Verification items for the finished model (mm, model axes). A direction names the side the tool comes from. Coordinates: 2 decimals unless noted, no trailing zeros. Order: outer loops, then holes, each group sorted by start corner. A loop starts at its lowest first (then second) coordinate and runs counter-clockwise, first axis right, second up. Notation, with made-up numbers: (4, 65) -> (50, 65) arc R35 ccw to (50, 102) -> close; hole circle Ø9 at (-26.75, 35). An arc over 180 degrees is marked (long way). Use CSV: the item, a comma, the result in double quotes. Start each with the question number.
1) Scan lines: line 1 along Z through (x, y) = (48.5, 22); line 2 along Y through (x, z) = (37, 275); line 3 along Z through (x, y) = (116.5, 240.5). Record each from-to range of solid material in increasing order.
2) Go/stop test with flat-tipped pins: pin 1 (5 mm diameter, centred on x = 3, z = 170.5, fed in from -Y); pin 2 (1 mm diameter, centred on x = 35, y = 323, fed in from -Z). Record where each tip stops, or that it passes through.
3) Sectioned sample at C-C on y = 319.5. Record the boundary of the cut face in (x, z).
4) Sectioned sample at D-D on x = 126.5. Record the boundary of the cut face in (y, z).
5) Tool access check on faces 1 (the flat face through (227, 7, 303)), 2 (the flat face through (15, 15, 324)), 3 (the flat face through (223, 32, 8)), 4 (the flat face through (113, 196, 15)). Record the directions out of +Z, -Z, +X, -X, +Y, -Y that give a thin tool (end or side, any length) a straight path to the whole face; none if there is none.
6) Sectioned sample at B-B on z = 138. Record the boundary of the cut face in (x, y).
7) Release check for a two-part mould opening along X. For faces 5 (the flat face through (0, 195, 185)), 6 (the flat face through (113, 395, 190)), 7 (the flat face through (4, 15, 336)) record: released by +X, released by -X, zero draft, split by the parting line, or undercut.
8) Sectioned sample at A-A on x = 50. Record the boundary of the cut face in (y, z), then the cut area to 3 significant figures.
from build123d import *

# Parameters (mm, degrees)
F0_W     = 230
F0_H     = 375
F1_DEPTH = 395
F2_SIZE  = 15
F4_DEPTH = 230.001
F6_DEPTH = 30
F8_DEPTH = 3


with BuildPart() as f1:
    # F0 (on Front) → F1 (new body)
    with BuildSketch(Plane.XZ):
        with Locations((115, 187.5)):
            Rectangle(F0_W, F0_H)
    extrude(amount=-F1_DEPTH)

    # F2
    f2_edges = [f1.edges().sort_by_distance(p)[0] for p in [
        (0, 197.5, 375),
        (0, 197.5, 0),
        (230, 197.5, 375),
        (230, 197.5, 0),
    ]]
    chamfer(f2_edges, length=F2_SIZE)

    # F3 (on face) → F4 (cut, through all)
    with BuildSketch(Plane(origin=(0, 0, 0), x_dir=(0, -1, 0), z_dir=(-1, 0, 0))):
        Polygon((-50, 0), (-65, 15), (-330, 15), (-345, 0), align=None)
        Polygon((-15, 80), (0, 65), (0, 310), (-15, 295), align=None)
    extrude(amount=-F4_DEPTH, mode=Mode.SUBTRACT)

    # F5 (on face) → F6 (cut)
    with BuildSketch(Plane.XZ):
        Polygon((15, 280), (15, 310), (4.8357864376, 310), (10, 289.3431457505), (10, 85.6568542495), (4, 61.6568542495), (4, 16.6568542495), (16.6568542495, 4), (115, 4), (213.3431457505, 4), (226, 16.6568542495), (226, 61.6568542495), (220, 85.6568542495), (220, 289.3431457505), (225.1642135624, 310), (215, 310), (215, 280), (205, 271.6090036882), (205, 103.3909963118), (215, 95), (215, 22), (203, 10), (163, 10), (154.6090036882, 20), (115, 20), (75.3909963118, 20), (67, 10), (27, 10), (15, 22), (15, 95), (25, 103.3909963118), (25, 271.6090036882), align=None)
        Polygon((15, 310), (15, 353), (27, 365), (115, 365), (203, 365), (215, 353), (215, 310), (225.1642135624, 310), (226, 313.3431457505), (226, 358.3431457505), (213.3431457505, 371), (115, 371), (16.6568542495, 371), (4, 358.3431457505), (4, 313.3431457505), (4.8357864376, 310), align=None)
    extrude(amount=-F6_DEPTH, mode=Mode.SUBTRACT)

    # F7 (on face) → F8 (cut)
    with BuildSketch(Plane.XZ.offset(-15)):
        Polygon((36, 262.3789077453), (25, 271.6090036882), (25, 103.3909963118), (36, 112.6210922547), align=None)
        Polygon((205, 103.3909963118), (205, 271.6090036882), (194, 262.3789077453), (194, 112.6210922547), align=None)
    extrude(amount=-F8_DEPTH, mode=Mode.SUBTRACT)


solid = f1.part
Answers follow:
1,line 1,"z = 0 to 4, 10 to 365, 371 to 375"
1,line 2,"y = 15 to 395"
1,line 3,"z = 15 to 375"
2,pin 1,"stops at y = 15"
2,pin 2,"stops at z = 15"
3,outline,"(0, 15) -> (230, 15) -> (230, 360) -> (215, 375) -> (15, 375) -> (0, 360) -> close"
4,outline,"(0, 0) -> (50, 0) -> (65, 15) -> (330, 15) -> (345, 0) -> (395, 0) -> (395, 375) -> (0, 375) -> (0, 371) -> (30, 371) -> (30, 365) -> (0, 365) -> (0, 310) -> (15, 295) -> (15, 80) -> (0, 65) -> (0, 20) -> (30, 20) -> (30, 4) -> (0, 4) -> close"
5,face 1,"+X, -X, -Y"
5,face 2,"-Y"
5,face 3,"-Z, +X, +Y, -Y"
5,face 4,"-Z, +X, -X"
6,outline,"(0, 15) -> (10, 15) -> (10, 30) -> (25, 30) -> (25, 18) -> (36, 18) -> (36, 15) -> (194, 15) -> (194, 18) -> (205, 18) -> (205, 30) -> (220, 30) -> (220, 15) -> (230, 15) -> (230, 395) -> (0, 395) -> close"
7,face 5,"released by -X"
7,face 6,"zero draft"
7,face 7,"undercut"
8,outline,"(0, 0) -> (50, 0) -> (65, 15) -> (330, 15) -> (345, 0) -> (395, 0) -> (395, 375) -> (0, 375) -> (0, 371) -> (30, 371) -> (30, 365) -> (0, 365) -> (0, 310) -> (15, 295) -> (15, 80) -> (0, 65) -> (0, 10) -> (30, 10) -> (30, 4) -> (0, 4) -> close"
8,area,"140,000 mm²"
